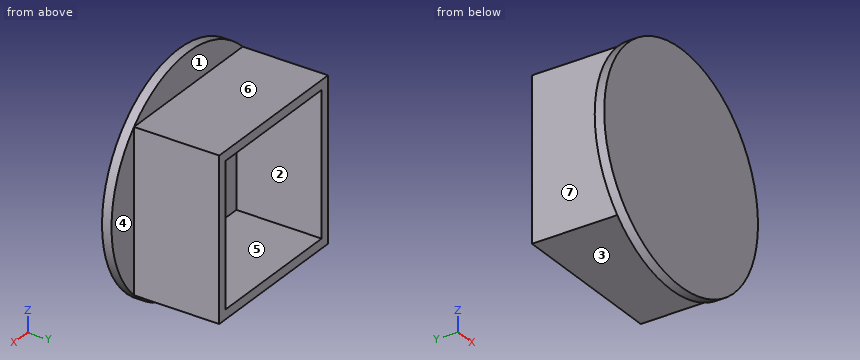
from build123d import *

# Parameters (mm, degrees)
SKETCH1_W           = 17
SKETCH1_H           = 17
SKETCH1_W_2         = 15
SKETCH1_H_2         = 15
EXTRUDE_THIN1_DEPTH = 10
SKETCH2_R           = 12.02081528
BOSS_EXTRUDE1_DEPTH = 1


with BuildPart() as part:
    # Sketch1 → Extrude-Thin1 (new body)
    with BuildSketch(Plane(origin=(0, 0, 0), x_dir=(1, 0, 0), z_dir=(0, 1, 0))):
        Rectangle(SKETCH1_W, SKETCH1_H)
        Rectangle(SKETCH1_W_2, SKETCH1_H_2, mode=Mode.SUBTRACT)
    extrude(amount=EXTRUDE_THIN1_DEPTH)

    # Sketch2 → Boss-Extrude1 (add)
    with BuildSketch(Plane(origin=(0, 0, 0), x_dir=(1, 0, 0), z_dir=(0, 1, 0))):
        Circle(SKETCH2_R)
    extrude(amount=BOSS_EXTRUDE1_DEPTH)


solid = part.part
Geometry check sheet. Reference: the model listing, model coordinates, mm. Face numbers are marked on the shaded views. A direction names the side the tool comes from. Round coordinates to 2 decimals unless told otherwise and drop trailing zeros. Loops run counter-clockwise (first coordinate to the right, second up) from the corner with the lowest first, then second, coordinate; pieces in that order, holes last.
Item 1: Cross-section at A-A on y = 9.5. Record the boundary of the cut face in (x, z), then the cut area to 3 significant figures.
Item 2: Gauge pin test, flat ends, axial feed: pin 1 (2.5 mm diameter, centred on x = -2, y = 5, fed in from +Z); pin 2 (1.1 mm diameter, centred on x = 10.5, z = 3, fed in from +Y); pin 3 (4 mm diameter, centred on x = -9.5, z = -1.5, fed in from +Y); pin 4 (2.5 mm diameter, centred on x = 3.5, y = 4.5, fed in from -Z). Record the tip position at first contact, or that the pin passes through.
Item 3: Access from +Z, -Z, +X, -X, +Y, -Y to the whole of each face (thin tool, end or side, straight path). Record for the marked faces 4, 5, 6 and 7.
Item 4: Cross-section at C-C on x = 0. Record the boundary of the cut face in (y, z).
Item 5: Mould release check, pull along Z, two halves, no side actions. Record for the marked faces 1, 2 and 3: pulls with the +Z half, pulls with the -Z half, needs draft (parallel to the pull), parting line crosses it, or undercut.
Item 6: Thickness scan on line 1 (Z direction, x = -4, y = 1.5); line 2 (Y direction, x = 4.25, z = -6.5). Record the ranges inside material, lowest first.
Item 7: Cross-section at B-B on z = 0. Record the boundary of the cut face in (x, y).
Item 8: Cross-section at D-D on x = -9.5. Record the boundary of the cut face in (y, z).
Answer sheet:
1. outline: (-8.5, -8.5) - (8.5, -8.5) - (8.5, 8.5) - (-8.5, 8.5) - close; hole (-7.5, -7.5) - (7.5, -7.5) - (7.5, 7.5) - (-7.5, 7.5) - close
1. area: 64.0 mm2
2. pin 1: stops at z = 8.5
2. pin 2: stops at y = 1
2. pin 3: stops at y = 10
2. pin 4: stops at z = -8.5
3. face 4: +Z, -Z, +X, +Y
3. face 5: +Y
3. face 6: +Z, +X, -X, +Y
3. face 7: +Z, -Z, -X, +Y
4. outline: (0, -12.02) - (1, -12.02) - (1, -8.5) - (10, -8.5) - (10, -7.5) - (1, -7.5) - (1, 7.5) - (10, 7.5) - (10, 8.5) - (1, 8.5) - (1, 12.02) - (0, 12.02) - close
5. face 1: needs draft
5. face 2: undercut
5. face 3: pulls with the -Z half
6. line 1: z = -8.5 to -7.5, 7.5 to 8.5
6. line 2: y = 0 to 1
7. outline: (-12.02, 0) - (12.02, 0) - (12.02, 1) - (8.5, 1) - (8.5, 10) - (7.5, 10) - (7.5, 1) - (-7.5, 1) - (-7.5, 10) - (-8.5, 10) - (-8.5, 1) - (-12.02, 1) - close
8. outline: (0, -7.37) - (1, -7.37) - (1, 7.37) - (0, 7.37) - close
